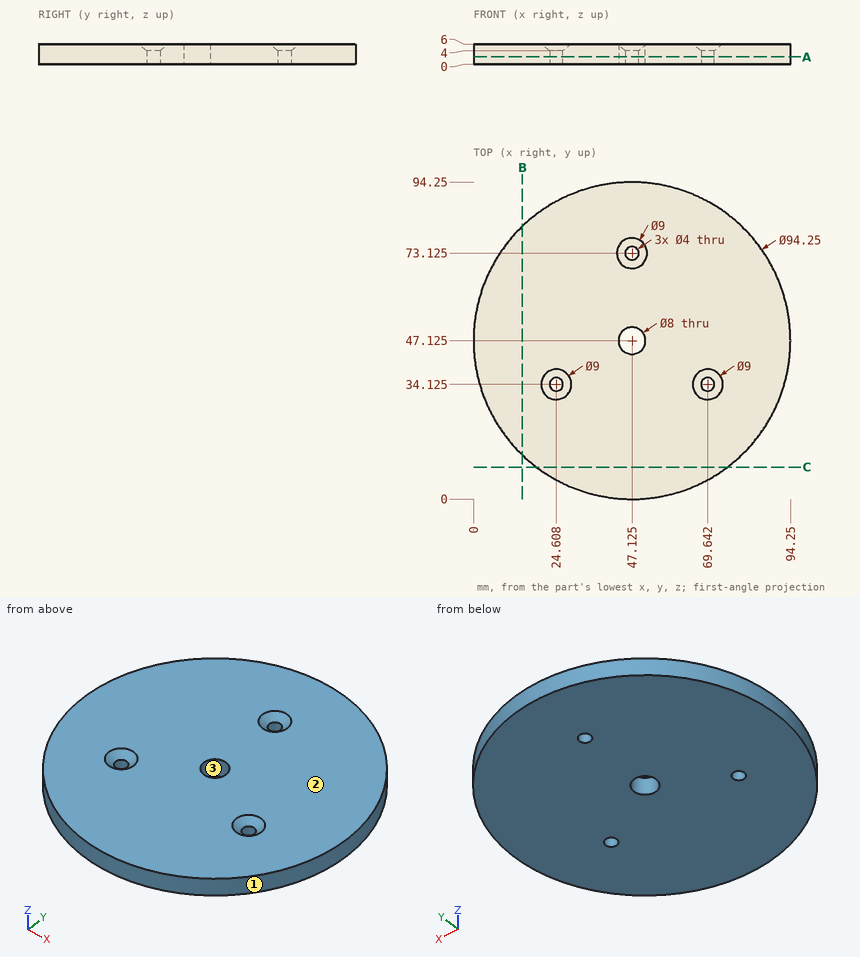
Answer from the drawing. Dimensions are ordinates in mm from the lowest x, y and z of the part. Coordinates: 2 decimals unless noted, no trailing zeros. Order: outer loops, then holes, each group sorted by start corner. A loop starts at its lowest first (then second) coordinate and runs counter-clockwise, first axis right, second up. Notation, with made-up numbers: (83.5, 19.5) - (108.5, 19.5) arc R14 cw to (108.5, 34.5) - close; hole circle Ø4 at (-21, -16.5). An arc over 180 degrees is marked (long way). Put each result on its own line as item: value. Start each with the question number.
1) Find the intervals of material crossed by line 1 (X direction, y = 45.5, z = 3.55); line 2 (X direction, y = 73, z = 3); line 3 (Y direction, x = 25, z = 4.75) (1 decimal), in increasing order. Write a range as from..to.
2) Find section B-B (x = 14.5). Give the vertices of the cut face in (y, z), plus the area to 3 significant figures.
3) Find section C-C (y = 9.5). Give the vertices of the cut face in (x, z).
4) For a pull along X with two mould halves and no side action, classify the marked faces 1, 2 and 3 as released by +X, released by -X, zero draft, split by the parting line, or undercut.
5) Flat-ended cylindrical pins translate along their axes: pin 1 (3 mm diameter, centred on x = 66, z = 2, fed in from +Y); pin 2 (3.5 mm diameter, centred on x = 24.61, y = 34.12, fed in from +Z); pin 3 (1 mm diameter, centred on x = 70.5, z = 4.5, fed in from -Y) (1 decimal); pin 4 (3 mm diameter, centred on x = 62, z = 3.5, fed in from -Y). Find the tip coordinate at first contact, or state that the pin passes through.
6) Find section A-A (z = 2.2). State how many separate pieces and enclosed holes the cut face has, plus the area to 3 significant figures.
Results list:
1. line 1: x = 0.03..43.47, 50.78..94.22
1. line 2: x = 7.74..45.13, 49.12..86.51
1. line 3: y = 5.5..31.2, 37..88.7
2. outline: (13.12, 0) - (81.13, 0) - (81.13, 6) - (13.12, 6) - close
2. area: 408 mm^2
3. outline: (18.75, 0) - (75.5, 0) - (75.5, 6) - (18.75, 6) - close
4. face 1: split by the parting line
4. face 2: zero draft
4. face 3: undercut
5. pin 1: stops at y = 90.93
5. pin 2: passes through
5. pin 3: stops at y = 5.9
5. pin 4: stops at y = 1.94
6. separate pieces: 1
6. enclosed holes: 4
6. area: 6,890 mm^2
